Source: CAD feature listing. Evaluate the final solid. Frame: model axes, mm. A direction names the side the tool comes from. Round coordinates to 2 decimals unless told otherwise and drop trailing zeros. Write each loop counter-clockwise with the first axis right and the second up, starting at its lowest first coordinate (ties: lowest second). Pieces come first, ordered by that corner, then holes. Notation, with made-up numbers: M 56,-32 L 92,-32 A15 ccw 92,-3 Z; hole C -32.75,38.5 d9. An arc over 180 degrees is marked long. Answer in a Markdown table with one row per item.
from build123d import *

# Parameters (mm, degrees)
BOSS_EXTRUDE1_DEPTH = 3.175
CUT_EXTRUDE2_REACH  = 132.832
SKETCH2_W           = 3
SKETCH2_H           = 6


with BuildPart() as part:
    # Sketch1 → Boss-Extrude1 (new body)
    with BuildSketch(Plane.XY):
        Polygon((0, 3.175), (15, 3.175), (18.175, 3.175), (18.175, 6.35), (15, 6.35), (15, 30.985), (18.175, 30.985), (18.175, 55.62), (15, 55.62), (15, 80.255), (18.175, 80.255), (18.175, 104.89), (15, 104.89), (15, 126.35), (18.175, 126.35), (18.175, 129.525), (15, 129.525), (0, 129.525), align=None)
    extrude(amount=BOSS_EXTRUDE1_DEPTH)

    # Sketch2 → Cut-Extrude2 (cut, up to next)
    with BuildSketch(Plane(origin=(0, 0, 0), x_dir=(-1, 0, 0), z_dir=(0, 0, -1)), mode=Mode.PRIVATE) as cut_extrude2_sk1:
        with Locations((-13.5, 66.35)):
            Rectangle(SKETCH2_W, SKETCH2_H)
    cut_extrude2_tool1 = extrude(cut_extrude2_sk1.sketch, amount=-CUT_EXTRUDE2_REACH, mode=Mode.PRIVATE) & part.part
    add(cut_extrude2_tool1.solids().sort_by_distance((13.5, 66.35, 0))[0], mode=Mode.SUBTRACT)


solid = part.part
Q1. Pull-direction query (Y, two-part tool) for faces 3 (the flat face through (9, 129.525, 2)), 4 (the flat face through (17, 126.35, 2)), 5 (the flat face through (7, 67, 0)); classes: pulls with the +Y half, pulls with the -Y half, needs draft (parallel to the pull), parting line crosses it, or undercut.
Solutions:
| item | result |
|---|---|
| face 3 | pulls with the +Y half |
| face 4 | undercut |
| face 5 | needs draft |
Q2. Section A-A (z = 0.65). Return loops of the section in (x, y) (3 decimals).
Solutions:
| item | result |
|---|---|
| outline | M 0,3.175 L 18.175,3.175 L 18.175,6.35 L 15,6.35 L 15,30.985 L 18.175,30.985 L 18.175,55.62 L 15,55.62 L 15,63.35 L 12,63.35 L 12,69.35 L 15,69.35 L 15,80.255 L 18.175,80.255 L 18.175,104.89 L 15,104.89 L 15,126.35 L 18.175,126.35 L 18.175,129.525 L 0,129.525 Z |
Q3. Material intervals for probe 1 along Y at (x, z) = (14, 1.25) (3 decimals); probe 2 along X at (y, z) = (72.5, 1.55), sorted ascending.
Solutions:
| item | result |
|---|---|
| probe 1 | y = 3.175 to 63.35, 69.35 to 129.525 |
| probe 2 | x = 0 to 15 |
Q4. Section B-B (y = 11). Return loops of the section in (x, z) (3 decimals).
Solutions:
| item | result |
|---|---|
| outline | M 0,0 L 15,0 L 15,3.175 L 0,3.175 Z |
Q5. Access query for faces 1 (the flat face through (14, 69.35, 2)), 2 (the flat face through (7, 67, 3.175)). Directions: +Z, -Z, +X, -X, +Y, -Y. A direction counts if a zero-diameter tool reaches every point of the face in a straight line with its end or side. Return the directions, or none.
Solutions:
| item | result |
|---|---|
| face 1 | +Z, -Z, +X |
| face 2 | +Z, +X, -X, +Y, -Y |
Q6. Contact query for flat-ended pins moving along their axis: pin 1 Ø1 at (y, z) = (65.5, 2) entering from +X; pin 2 Ø1.5 at (y, z) = (18.5, 1) entering from +X. Output: stop coordinate, or through.
Solutions:
| item | result |
|---|---|
| pin 1 | stops at x = 12 |
| pin 2 | stops at x = 15 |
